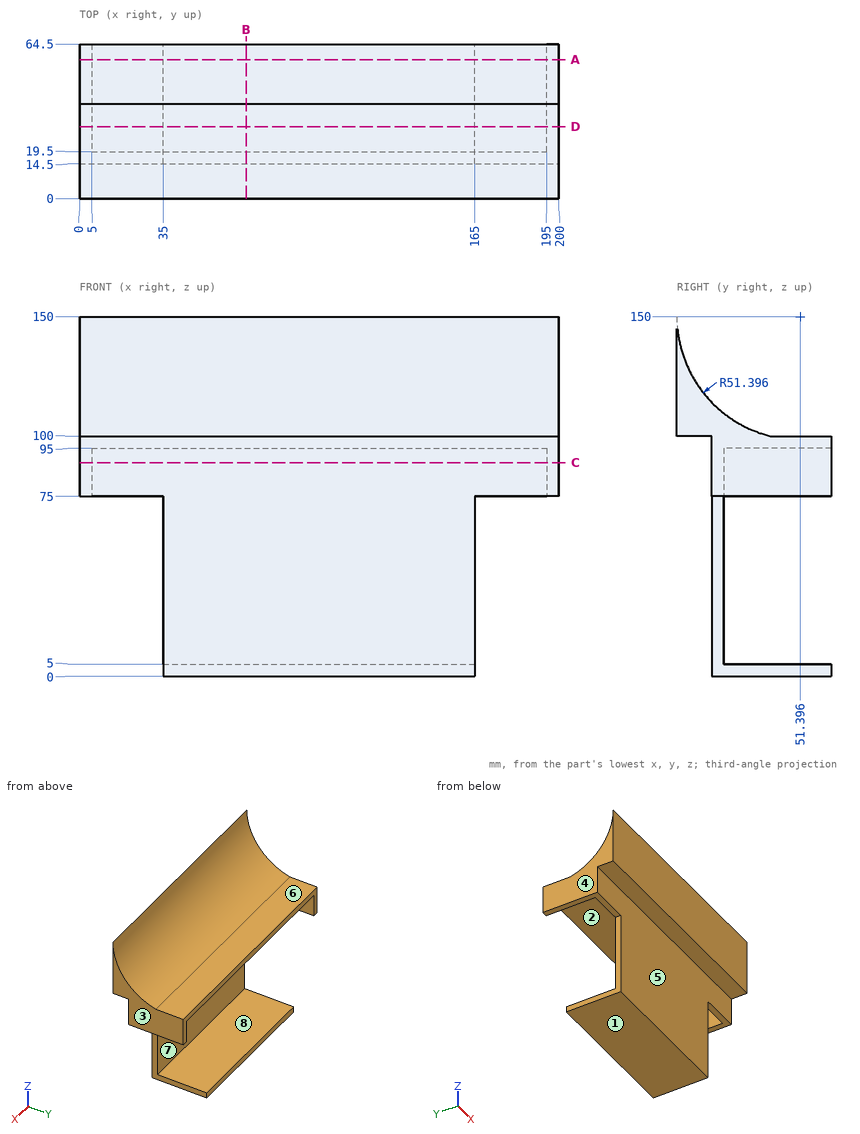
Source: three-view drawing plus pictorial views. Frame: mm from the lowest corner of the part. A direction names the side the tool comes from. Round coordinates to 2 decimals unless told otherwise and drop trailing zeros. Order: outer loops, then holes, each group sorted by start corner. A loop starts at its lowest first (then second) coordinate and runs counter-clockwise, first axis right, second up. Notation, with made-up numbers: (-32.5, -20) -> (-3.5, -20) arc R32 ccw to (-3.5, 8) -> close; hole circle Ø5 at (-9.5, 27.5). An arc over 180 degrees is marked (long way). Use one line per item in the form item = value. Start each with the question number.
1. Line query: probe 1 along Z at (x, y) = (15, 42); probe 2 along Y at (x, z) = (100.5, 29); probe 3 along Z at (x, y) = (156, 52). Output: solid intervals per line, ascending.
2. Reachability of the marked faces 5, 6, 7 and 8 from +Z, -Z, +X, -X, +Y, -Y: full face, straight path, thin tool, end or side. Return the list, or none.
3. Cut plane C-C (z = 89). Return the cut outline in (x, y).
4. Draft query along X for the marked faces 1, 2, 3 and 4. Return one class per face: pulls with the +X half, pulls with the -X half, needs draft (parallel to the pull), parting line crosses it, or undercut.
5. Cut plane A-A (y = 58). Return the cut outline in (x, z).
6. Pin query (flat end, axial travel): pin 1 Ø2 at (y, z) = (16.5, 26) entering from -X; pin 2 Ø8 at (x, z) = (87.5, 17.5) entering from +Y; pin 3 Ø1 at (x, z) = (65.5, 46) entering from -Y. Return the tip coordinate at first contact, or that it passes through.
7. Cut plane D-D (y = 30). Return the cut outline in (x, z), then the cut area to 3 significant figures.
8. Cut plane B-B (x = 69.5). Return the cut outline in (y, z) (1 decimal).
Solution:
q1.probe_1 = 95 to 100
q1.probe_2 = 14.5 to 19.5
q1.probe_3 = 0 to 5, 95 to 100
q2.face_5 = -Z, +X, -X, -Y
q2.face_6 = +Z, +X, -X, +Y
q2.face_7 = +Y
q2.face_8 = +X, -X, +Y
q3.outline = (0, 14.5) -> (200, 14.5) -> (200, 64.5) -> (195, 64.5) -> (195, 19.5) -> (5, 19.5) -> (5, 64.5) -> (0, 64.5) -> close
q4.face_1 = needs draft
q4.face_2 = undercut
q4.face_3 = pulls with the +X half
q4.face_4 = pulls with the -X half
q5.outline = (0, 75) -> (5, 75) -> (5, 95) -> (195, 95) -> (195, 75) -> (200, 75) -> (200, 100) -> (0, 100) -> close; (35, 0) -> (165, 0) -> (165, 5) -> (35, 5) -> close
q6.pin_1 = 35
q6.pin_2 = 19.5
q6.pin_3 = 14.5
q7.outline = (0, 75) -> (5, 75) -> (5, 95) -> (195, 95) -> (195, 75) -> (200, 75) -> (200, 103.27) -> (0, 103.27) -> close; (35, 0) -> (165, 0) -> (165, 5) -> (35, 5) -> close
q7.area = 2,500 mm^2
q8.outline = (0, 100) -> (14.5, 100) -> (14.5, 0) -> (64.5, 0) -> (64.5, 5) -> (19.5, 5) -> (19.5, 95) -> (64.5, 95) -> (64.5, 100) -> (39.5, 100) arc R51.4 cw to (0, 150) -> close
